Can you work these out from the model? Positions are in its coordinate system, mm. Face numbers are marked on the shaded views. Coordinates: 2 decimals unless noted, no trailing zeros. Loops run counter-clockwise (first coordinate to the right, second up) from the corner with the lowest first, then second, coordinate; pieces in that order, holes last.
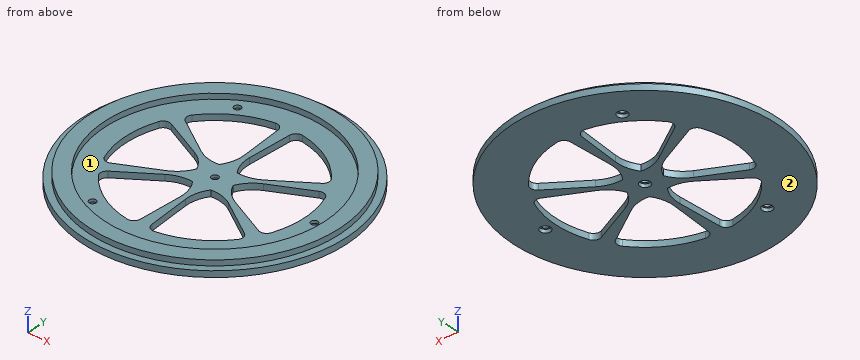
```python
from build123d import *

# Parameters (mm, degrees)
SKETCH_1_R                       = 38.5
EXTRUDE_1_DEPTH                  = 2
SKETCH_2_OUTSIDE_W               = 100.782
SKETCH_2_OUTSIDE_H               = 100.782
SKETCH_2_OUTSIDE_R               = 36.5
SKETCH_2_OUTSIDE_R_2             = 32.1
CUT_EXTRUDE_1_DEPTH              = 0.2
EXTRUDE_START                    = 1.4
SKETCH_2_2_R                     = 36.5
SKETCH_2_2_R_2                   = 32.1
EXTRUDE_2_DEPTH                  = 1.4
SKETCH_3_R                       = 26.1
CUT_EXTRUDE_2_DEPTH              = 55.47696761
SKETCH_3_3_R                     = 5
EXTRUDE_3_DEPTH                  = 1.8
EXTRUDE_4_DEPTH                  = 1.8
FILLET_1_R                       = 2
PATTERN_CIRCULAR_1_COUNT         = 6
FILLET_1_OF_PATTERN_CIRCULAR_1_R = 2
FILLET_2_R                       = 10
SKETCH_4_R                       = 1
CUT_EXTRUDE_3_DEPTH              = 55.47696761
CUT_EXTRUDE_START                = -1.8
SKETCH_4_3_R                     = 1.5
CUT_EXTRUDE_4_DEPTH              = 1


with BuildPart() as part:
    # Sketch 1 → Extrude 1 (new body)
    with BuildSketch(Plane.XY):
        Circle(SKETCH_1_R)
    extrude(amount=EXTRUDE_1_DEPTH)

    # Sketch 2 outside → Cut-Extrude 1 (cut)
    # profile 1 of 2: a face of its own
    with BuildSketch(Plane.XY.offset(2)):
        Rectangle(SKETCH_2_OUTSIDE_W, SKETCH_2_OUTSIDE_H)
        Circle(SKETCH_2_OUTSIDE_R, mode=Mode.SUBTRACT)
    # profile 2 of 2: a face of its own
    with BuildSketch(Plane.XY.offset(2)):
        Circle(SKETCH_2_OUTSIDE_R_2)
    extrude(amount=-CUT_EXTRUDE_1_DEPTH, mode=Mode.SUBTRACT)

    # Sketch 2_2 → Extrude 2 (add)
    with BuildSketch(Plane.XY.offset(2).offset(EXTRUDE_START)):
        Circle(SKETCH_2_2_R)
        Circle(SKETCH_2_2_R_2, mode=Mode.SUBTRACT)
    extrude(amount=-EXTRUDE_2_DEPTH)

    # Sketch 3 → Cut-Extrude 2 (cut, through all)
    with BuildSketch(Plane.XY.offset(1.8)):
        Circle(SKETCH_3_R)
    extrude(amount=-CUT_EXTRUDE_2_DEPTH, mode=Mode.SUBTRACT)



with BuildPart() as body_2:
    # Sketch 3_3 → Extrude 3 (new, through all)
    with BuildSketch(Plane.XY.offset(1.8)):
        Circle(SKETCH_3_3_R)
    extrude(amount=-EXTRUDE_3_DEPTH)


with BuildPart() as part_1:
    add(part.part)

    add(body_2.part)  # Extrude 4 merges body 2
    # Sketch 3_4 → Extrude 4 (add, through all)
    with BuildSketch(Plane.XY.offset(1.8)):
        with BuildLine():
            ThreePointArc((1.820643965, 26.036421712), (0, 26.1), (-1.820643965, 26.036421712))
            Line((-1.820643965, 26.036421712), (-0.348782369, 4.987820251))
            ThreePointArc((-0.348782369, 4.987820251), (0, 5), (0.348782369, 4.987820251))
            Line((0.348782369, 4.987820251), (1.820643965, 26.036421712))
        make_face()
    extrude_4 = extrude(amount=-EXTRUDE_4_DEPTH)

    # Fillet 1
    fillet_1_edges = [part_1.edges().sort_by_distance(p)[0] for p in [
        (-1.820643965, 26.036421712, 0.9),
        (1.820643965, 26.036421712, 0.9),
    ]]
    fillet(fillet_1_edges, radius=FILLET_1_R)

    # Pattern Circular 1: Extrude 4 ×6 about axis
    pattern_circular_1_axis = Axis((0, 0, 0), (0, 0, 1))
    for i in range(1, PATTERN_CIRCULAR_1_COUNT):
        add(extrude_4.rotate(pattern_circular_1_axis, i * 360 / PATTERN_CIRCULAR_1_COUNT))

    # Fillet 1 of Pattern Circular 1
    fillet_1_of_pattern_circular_1_edges = [part_1.edges().sort_by_distance(p)[0] for p in [
        (-23.458524608, 11.441486931, 0.9),
        (-21.637880644, 14.594934781, 0.9),
        (-21.637880644, -14.594934781, 0.9),
        (-23.458524608, -11.441486931, 0.9),
        (1.820643965, -26.036421712, 0.9),
        (-1.820643965, -26.036421712, 0.9),
        (23.458524608, -11.441486931, 0.9),
        (21.637880644, -14.594934781, 0.9),
        (21.637880644, 14.594934781, 0.9),
        (23.458524608, 11.441486931, 0.9),
    ]]
    fillet(fillet_1_of_pattern_circular_1_edges, radius=FILLET_1_OF_PATTERN_CIRCULAR_1_R)

    # Fillet 2
    # the kernel refuses this fillet: 10 mm, written as the material it adds along each edge
    with BuildSketch(Plane(origin=(4.493970231, -2.191855734, 1.8), x_dir=(0.8987940462991597, -0.4383711467890922, 0), z_dir=(0, 0, -1)), Plane(origin=(0.348782369, -4.987820251, 1.8), x_dir=(0.06975647374410966, -0.9975640502598253, 0), z_dir=(0, 0, -1)), Plane(origin=(-4.145187863, -2.795964517, 1.8), x_dir=(-0.8290375725550504, -0.5591929034707338, 0), z_dir=(0, 0, -1)), Plane(origin=(-4.493970231, 2.191855734, 1.8), x_dir=(-0.8987940462991602, 0.4383711467890914, 0), z_dir=(0, 0, -1)), Plane(origin=(-0.348782369, 4.987820251, 1.8), x_dir=(-0.06975647374410977, 0.9975640502598253, 0), z_dir=(0, 0, -1)), Plane(origin=(4.145187863, 2.795964517, 1.8), x_dir=(0.8290375725550504, 0.5591929034707338, 0), z_dir=(0, 0, -1))) as fillet_2_piece_1:
        with BuildLine():
            CenterArc((6.180339887, -10), FILLET_2_R, 90, 48.189685104)
            ThreePointArc((-1.273220038, -3.333333333), (-0.329138205, -1.784110449), (0, 0))
            Line((0, 0), (6.180339887, 0))
        make_face()
    extrude(amount=1.8)
    with BuildSketch(Plane(origin=(4.493970231, 2.191855734, 1.8), x_dir=(0.8987940462991614, 0.4383711467890888, 0), z_dir=(0, 0, -1)), Plane(origin=(4.145187863, -2.795964517, 1.8), x_dir=(0.8290375725550488, -0.5591929034707364, 0), z_dir=(0, 0, -1)), Plane(origin=(-0.348782369, -4.987820251, 1.8), x_dir=(-0.06975647374411244, -0.9975640502598251, 0), z_dir=(0, 0, -1)), Plane(origin=(-4.493970231, -2.191855734, 1.8), x_dir=(-0.8987940462991615, -0.43837114678908895, 0), z_dir=(0, 0, -1)), Plane(origin=(-4.145187863, 2.795964517, 1.8), x_dir=(-0.8290375725550488, 0.5591929034707362, 0), z_dir=(0, 0, -1)), Plane(origin=(0.348782369, 4.987820251, 1.8), x_dir=(0.06975647374411233, 0.9975640502598251, 0), z_dir=(0, 0, -1))) as fillet_2_piece_2:
        with BuildLine():
            CenterArc((6.180339887, 10), FILLET_2_R, 221.810314896, 48.189685104)
            ThreePointArc((-1.273220038, 3.333333333), (-0.329138205, 1.784110449), (0, 0))
            Line((0, 0), (6.180339887, 0))
        make_face()
    extrude(amount=1.8)

    # Sketch 4 → Cut-Extrude 3 (cut, through all)
    with BuildSketch(Plane.XY.offset(1.8)):
        with Locations((-14.55, 25.20133925)):
            Circle(SKETCH_4_R)
        Circle(SKETCH_4_R)
        with Locations((29.1, 0)):
            Circle(SKETCH_4_R)
        with Locations((-14.55, -25.20133925)):
            Circle(SKETCH_4_R)
    extrude(amount=-CUT_EXTRUDE_3_DEPTH, mode=Mode.SUBTRACT)

    # Sketch 4_3 → Cut-Extrude 4 (cut)
    with BuildSketch(Plane.XY.offset(1.8).offset(CUT_EXTRUDE_START)):
        with Locations((-14.55, 25.20133925)):
            Circle(SKETCH_4_3_R)
        with Locations((29.1, 0)):
            Circle(SKETCH_4_3_R)
        with Locations((-14.55, -25.20133925)):
            Circle(SKETCH_4_3_R)
        Circle(SKETCH_4_3_R)
    extrude(amount=CUT_EXTRUDE_4_DEPTH, mode=Mode.SUBTRACT)


solid = part_1.part
```
(1) I'm going to push flat-ended pins straight in: pin 1 (2.5 mm diameter, centred on x = -14.55, y = -25.2, fed in from +Z); pin 2 (2.5 mm diameter, centred on x = -14.55, y = 25.2, fed in from -Z); pin 3 (6 mm diameter, centred on x = 10.5, y = 20, fed in from -Z). Where does each tip first touch, or does it pass through?
Check values:
pin 1: stops at z = 1.8
pin 2: stops at z = 1
pin 3: passes through
(2) I want a section at C-C on y = -29. Write out the boundary of the cut face in (x, z), then the cut area to 3 significant figures.
Check values:
outline: (-25.32, 0) - (25.32, 0) - (25.32, 1.8) - (22.16, 1.8) - (22.16, 3.4) - (13.76, 3.4) - (13.76, 1.8) - (-13.76, 1.8) - (-13.76, 3.4) - (-22.16, 3.4) - (-22.16, 1.8) - (-25.32, 1.8) - close
area: 118 mm2
(3) I want a section at D-D on x = -14.55. State how many separate pieces and enclosed holes the cut face has, then the cut area to 3 significant figures.
Check values:
separate pieces: 6
enclosed holes: 0
area: 66.5 mm2
(4) I want a section at B-B on x = 29.1. Write out the boundary of the cut face in (y, z), then the cut area to 3 significant figures.
Check values:
outline: (-25.21, 0) - (-1.5, 0) - (-1.5, 1) - (-1, 1) - (-1, 1.8) - (-13.55, 1.8) - (-13.55, 3.4) - (-22.03, 3.4) - (-22.03, 1.8) - (-25.21, 1.8) - close; (1, 1) - (1.5, 1) - (1.5, 0) - (25.21, 0) - (25.21, 1.8) - (22.03, 1.8) - (22.03, 3.4) - (13.55, 3.4) - (13.55, 1.8) - (1, 1.8) - close
area: 113 mm2
(5) I want a section at A-A on y = -21. Write out the boundary of the cut face in (x, z).
Check values:
outline: (-32.27, 0) - (-15.5, 0) - (-15.5, 1.8) - (-24.28, 1.8) - (-24.28, 3.4) - (-29.85, 3.4) - (-29.85, 1.8) - (-32.27, 1.8) - close; (-1.47, 0) - (1.47, 0) - (1.47, 1.8) - (-1.47, 1.8) - close; (15.5, 0) - (32.27, 0) - (32.27, 1.8) - (29.85, 1.8) - (29.85, 3.4) - (24.28, 3.4) - (24.28, 1.8) - (15.5, 1.8) - close
(6) If we mould it in two halves opening along Y, with no side actions, what happens to the marked faces 1 and 2? For each: released by +Y, released by -Y, zero draft, split by the parting line, or undercut.
Check values:
face 1: undercut
face 2: zero draft
(7) If I drill on probe 1 along Y at (x, z) = (-14.55, 1.35); probe 2 along Y at (x, z) = (0, 1.5); probe 3 along Y at (x, z) = (3, 0.6), over which ranges is the centre line in solid material (lowest first)?
Check values:
probe 1: y = -35.64 to -26.2, -24.2 to -21.67, -9.81 to -7.1, 7.1 to 9.81, 21.67 to 24.2, 26.2 to 35.64
probe 2: y = -38.5 to -1, 1 to 38.5
probe 3: y = -38.38 to -25.7, -4.57 to 4.57, 25.7 to 38.38
